from build123d import *

# Parameters (mm, degrees)
SALIENTE_EXTRUIR1_DEPTH      = 40
SALIENTE_EXTRUIR1_DEPTH_BACK = 40
CROQUIS2_R                   = 17
CORTAR_EXTRUIR1_DEPTH        = 2
CORTAR_EXTRUIR2_REACH        = 118.486
CROQUIS5_R                   = 13
CROQUIS6_R                   = 15
CORTAR_EXTRUIR3_DEPTH        = 20
CORTAR_EXTRUIR4_START        = -20
CROQUIS7_R                   = 15
CORTAR_EXTRUIR4_DEPTH        = 20
CORTAR_EXTRUIR6_REACH        = 105.562
CROQUIS8_R                   = 5.5
CROQUIS9_R                   = 4
CORTAR_EXTRUIR7_DEPTH        = 30
CROQUIS10_R                  = 3
CORTAR_EXTRUIR8_DEPTH        = 25


with BuildPart() as part:
    # Croquis1 → Saliente-Extruir1 (new, two sides: drawn at the far end of the back side and taken through both)
    with BuildSketch(Plane.XY.offset(-SALIENTE_EXTRUIR1_DEPTH_BACK)):
        Polygon((65, 0), (-65, 0), (-65, 20), (-43, 20), (-43, 90), (43, 90), (43, 20), (65, 20), align=None)
    extrude(amount=SALIENTE_EXTRUIR1_DEPTH + SALIENTE_EXTRUIR1_DEPTH_BACK)

    # Croquis2 → Cortar-Extruir1 (cut)
    with BuildSketch(Plane(origin=(0, 90, 0), x_dir=(1, 0, 0), z_dir=(0, 1, 0))):
        with Locations(Location((0, 0, 0), (0, 0, 270))):
            Circle(CROQUIS2_R)
    extrude(amount=-CORTAR_EXTRUIR1_DEPTH, mode=Mode.SUBTRACT)

    # Croquis4 → Cortar-Revoluci_n2 (revolve, cut)
    with BuildSketch(Plane.XY, mode=Mode.PRIVATE) as cortar_revoluci_n2_sk:
        Polygon((-35, 90), (-75.552498824, 49.447501176), (-75.552498824, 90), align=None)
    revolve(cortar_revoluci_n2_sk.sketch.rotate(Axis((0, 0, 0), (0, -1, 0)), 137.070029202), axis=Axis((0, 0, 0), (0, -1, 0)), mode=Mode.SUBTRACT)

    # Croquis5 → Cortar-Extruir2 (cut, up to next)
    with BuildSketch(Plane(origin=(0, 88, 0), x_dir=(1, 0, 0), z_dir=(0, 1, 0)), mode=Mode.PRIVATE) as cortar_extruir2_sk1:
        with Locations(Location((0, 0, 0), (0, 0, 270))):
            Circle(CROQUIS5_R)
    cortar_extruir2_tool1 = extrude(cortar_extruir2_sk1.sketch, amount=-CORTAR_EXTRUIR2_REACH, mode=Mode.PRIVATE) & part.part
    add(cortar_extruir2_tool1.solids().sort_by_distance((0, 88, 0))[0], mode=Mode.SUBTRACT)

    # Croquis6 → Cortar-Extruir3 (cut)
    with BuildSketch(Plane(origin=(0, 88, 0), x_dir=(1, 0, 0), z_dir=(0, 1, 0))):
        with Locations(Location((0, 0, 0), (0, 0, 270))):
            Circle(CROQUIS6_R)
    extrude(amount=-CORTAR_EXTRUIR3_DEPTH, mode=Mode.SUBTRACT)

    # Croquis7 → Cortar-Extruir4 (cut)
    with BuildSketch(Plane.XZ.offset(CORTAR_EXTRUIR4_START)):
        with Locations(Location((0, 0, 0), (0, 0, 90))):
            Circle(CROQUIS7_R)
    extrude(amount=CORTAR_EXTRUIR4_DEPTH, mode=Mode.SUBTRACT)

    # Croquis8 → Cortar-Extruir6 (cut, up to next)
    with BuildSketch(Plane(origin=(0, 20, 0), x_dir=(1, 0, 0), z_dir=(0, 1, 0)), mode=Mode.PRIVATE) as cortar_extruir6_sk1:
        with Locations(Location((-55, 30, 0), (0, 0, 270))):
            Circle(CROQUIS8_R)
    cortar_extruir6_tool1 = extrude(cortar_extruir6_sk1.sketch, amount=-CORTAR_EXTRUIR6_REACH, mode=Mode.PRIVATE) & part.part
    # Croquis8 → Cortar-Extruir6 (cut, up to next)
    with BuildSketch(Plane(origin=(0, 20, 0), x_dir=(1, 0, 0), z_dir=(0, 1, 0)), mode=Mode.PRIVATE) as cortar_extruir6_sk2:
        with Locations(Location((-55, -30, 0), (0, 0, 270))):
            Circle(CROQUIS8_R)
    cortar_extruir6_tool2 = extrude(cortar_extruir6_sk2.sketch, amount=-CORTAR_EXTRUIR6_REACH, mode=Mode.PRIVATE) & part.part
    # Croquis8 → Cortar-Extruir6 (cut, up to next)
    with BuildSketch(Plane(origin=(0, 20, 0), x_dir=(1, 0, 0), z_dir=(0, 1, 0)), mode=Mode.PRIVATE) as cortar_extruir6_sk3:
        with Locations(Location((55, 30, 0), (0, 0, 270))):
            Circle(CROQUIS8_R)
    cortar_extruir6_tool3 = extrude(cortar_extruir6_sk3.sketch, amount=-CORTAR_EXTRUIR6_REACH, mode=Mode.PRIVATE) & part.part
    # Croquis8 → Cortar-Extruir6 (cut, up to next)
    with BuildSketch(Plane(origin=(0, 20, 0), x_dir=(1, 0, 0), z_dir=(0, 1, 0)), mode=Mode.PRIVATE) as cortar_extruir6_sk4:
        with Locations(Location((55, -30, 0), (0, 0, 270))):
            Circle(CROQUIS8_R)
    cortar_extruir6_tool4 = extrude(cortar_extruir6_sk4.sketch, amount=-CORTAR_EXTRUIR6_REACH, mode=Mode.PRIVATE) & part.part
    add(cortar_extruir6_tool1.solids().sort_by_distance((-55, 20, -30))[0], mode=Mode.SUBTRACT)
    add(cortar_extruir6_tool2.solids().sort_by_distance((-55, 20, 30))[0], mode=Mode.SUBTRACT)
    add(cortar_extruir6_tool3.solids().sort_by_distance((55, 20, -30))[0], mode=Mode.SUBTRACT)
    add(cortar_extruir6_tool4.solids().sort_by_distance((55, 20, 30))[0], mode=Mode.SUBTRACT)

    # Croquis9 → Cortar-Extruir7 (cut)
    with BuildSketch(Plane.XY.offset(40)):
        with Locations((-20, 63)):
            Circle(CROQUIS9_R)
        with Locations((20, 63)):
            Circle(CROQUIS9_R)
        with Locations((20, 15)):
            Circle(CROQUIS9_R)
        with Locations((-20, 15)):
            Circle(CROQUIS9_R)
    extrude(amount=-CORTAR_EXTRUIR7_DEPTH, mode=Mode.SUBTRACT)

    # Croquis10 → Cortar-Extruir8 (cut)
    with BuildSketch(Plane(origin=(0, 90, 0), x_dir=(1, 0, 0), z_dir=(0, 1, 0))):
        with Locations(Location((0, 26.5, 0), (0, 0, 180))):
            Circle(CROQUIS10_R)
        with Locations(Location((26.5, 0, 0), (0, 0, 180))):
            Circle(CROQUIS10_R)
        with Locations(Location((0, -26.5, 0), (0, 0, 180))):
            Circle(CROQUIS10_R)
        with Locations(Location((-26.5, 0, 0), (0, 0, 180))):
            Circle(CROQUIS10_R)
    extrude(amount=-CORTAR_EXTRUIR8_DEPTH, mode=Mode.SUBTRACT)


solid = part.part
Design review of the part built by this model. Coordinates are the model's own, in mm. A direction names the side the tool comes from. Coordinates: 2 decimals unless noted, no trailing zeros. Loops run counter-clockwise (first coordinate to the right, second up) from the corner with the lowest first, then second, coordinate; pieces in that order, holes last. Notation, with made-up numbers: M 10.5,72.25 L 40.5,72.25 A25 cw 40.5,101.25 Z; hole C 63.25,35 d11. An arc over 180 degrees is marked long. Use one line per item in the form item = value.
(1) Consider section B-B (y = 73.5). Write out the cut boundary in (x, z).
Return value:
outline = M -43,-28.34 A51.5 ccw -32.44,-40 L 32.44,-40 A51.5 ccw 43,-28.34 L 43,28.34 A51.5 ccw 32.44,40 L -32.44,40 A51.5 ccw -43,28.34 Z; hole C -26.5,0 d6; hole C 0,0 d30; hole C 0,-26.5 d6; hole C 0,26.5 d6; hole C 26.5,0 d6
(2) Consider section C-C (z = 26.5). Give the number of separate pieces and of enclosed holes in the cut face, and give its area (3 significant figures).
Return value:
separate_pieces = 3
enclosed_holes = 4
area = 7,630 mm2
(3) For line 1 along X through (y, z) = (6, 30); line 2 along Y through (x, z) = (20, 32); line 3 along X through (y, z) = (13.5, -26.5), list the stretches that pass through material, from the lowest coordinate up. Write a range as from..to.
Return value:
line_1 = -65..-60.5, -49.5..49.5, 60.5..65
line_2 = 0..11, 19..59, 67..87.26
line_3 = -65..-59.24, -50.76..50.76, 59.24..65
(4) Consider section A-A (x = -55). Write out the cut boundary in (y, z), and give its area (3 significant figures).
Return value:
outline = M 0,-40 L 20,-40 L 20,-35.5 L 0,-35.5 Z; M 0,-24.5 L 20,-24.5 L 20,24.5 L 0,24.5 Z; M 0,35.5 L 20,35.5 L 20,40 L 0,40 Z
area = 1,160 mm2
(5) For faces 4 (the face through (-43, 51, -1)), 5 (the face through (13.4, 68, -0.1)), 6 (the face through (43, 51, -1)), 7 (the face through (-20.867, 59.095, 25.21)), list the 3-axis set-ups (+Z, -Z, +X, -X, +Y, -Y) from which the entire face can be reached by the end or side of a thin tool; tool diameter is ignored.
Return value:
face_4 = +Z, -Z, -X, +Y
face_5 = +Y
face_6 = +Z, -Z, +X, +Y
face_7 = +Z
(6) Draft analysis for pull direction Z (two halves, no side actions). For faces 1 (the face through (-13.4, 20, -0.1)), 2 (the face through (-25.59, 88.52, 26)), 3 (the face through (-65, 10, -1)), state which applies: pulls with the +Z half, pulls with the -Z half, needs draft (parallel to the pull), parting line crosses it, or undercut.
Return value:
face_1 = undercut
face_2 = parting line crosses it
face_3 = needs draft
(7) Clearance check with flat-ended pins moving along their axes: P1, Ø10, axis at x = 3, z = 1.5, coming from the +Y side; P2, Ø3, axis at x = -26.5, z = 1, coming from the +Y side; P3, Ø4, axis at y = 26.5, z = -21, coming from the +X side; P4, Ø24, axis at x = 55.5, z = -7.5, coming from the +Y side. State where each tip first meets the part, or that it passes through.
Return value:
P1 = through
P2 = 65
P3 = 43
P4 = 20
(8) Consider section D-D (y = 44). Write out the cut boundary in (x, z).
Return value:
outline = M -43,-40 L 43,-40 L 43,40 L -43,40 Z; hole C 0,0 d26
